Here's how the part is built. I have some questions about the finished solid (model axes, mm). Face numbers are marked on the shaded views. A direction names the side the tool comes from. Give positions to 0.01 mm unless a question says otherwise; leave off trailing zeros. Write each loop counter-clockwise with the first axis right and the second up, starting at its lowest first coordinate (ties: lowest second). Pieces come first, ordered by that corner, then holes. Notation, with made-up numbers: (-27.5, 60.5) - (27.5, 60.5) arc R21 cw to (27.5, 96.5) - close; hole circle Ø5 at (-4, -33.5). An arc over 180 degrees is marked (long way). Use a Markdown table: item, result.
```python
from build123d import *

# Parameters (mm, degrees)
SKETCH2_W           = 115
SKETCH2_H           = 95
BOSS_EXTRUDE1_DEPTH = 5
SKETCH3_W           = 62
SKETCH3_H           = 4
BOSS_EXTRUDE2_DEPTH = 44
RIB1_REACH          = 135.725
SKETCH5_WALL_W      = 295.338836254
SKETCH5_WALL_H      = 8
RIB2_START          = -8
RIB2_DEPTH          = 8
RIB6_REACH          = 135.725
SKETCH7_WALL_W      = 295.32906057
SKETCH7_WALL_H      = 8
BOSS_EXTRUDE3_DEPTH = 8
SKETCH11_R          = 13
SKETCH11_R_2        = 2.1
CUT_EXTRUDE1_DEPTH  = 4
SKETCH12_R          = 13
SKETCH12_R_2        = 2.1
CUT_EXTRUDE2_DEPTH  = 4
SKETCH13_R          = 2.6
CUT_EXTRUDE3_DEPTH  = 5


# Read off the part's stored shape, not the designer's step: Rib2
with BuildPart() as part:
    # Sketch2 → Boss-Extrude1 (new body)
    with BuildSketch(Plane(origin=(0, 0, 0), x_dir=(1, 0, 0), z_dir=(0, 1, 0))):
        Rectangle(SKETCH2_W, SKETCH2_H)
    extrude(amount=BOSS_EXTRUDE1_DEPTH)

    # Sketch3 → Boss-Extrude2 (add)
    with BuildSketch(Plane(origin=(0, 5, 0), x_dir=(1, 0, 0), z_dir=(0, 1, 0))):
        with Locations((-26.5, 45.5)):
            Rectangle(SKETCH3_W, SKETCH3_H)
        with Locations((26.5, -45.5)):
            Rectangle(SKETCH3_W, SKETCH3_H)
    extrude(amount=BOSS_EXTRUDE2_DEPTH)

    # Sketch5 wall → Rib1 (add, up to next)
    with BuildSketch(Plane(origin=(57.5, 14.153417974, 34.346582025), x_dir=(0, -0.707106781187, -0.707106781187), z_dir=(0, 0.707106781187, -0.707106781187)), mode=Mode.PRIVATE) as rib1_sk1:
        with Locations((0, 4)):
            Rectangle(SKETCH5_WALL_W, SKETCH5_WALL_H)
    rib1_tool1 = extrude(rib1_sk1.sketch, amount=-RIB1_REACH, mode=Mode.PRIVATE) - part.part
    add(rib1_tool1.solids().sort_by_distance((57.5, 14.153417974, 34.346582025))[0])

    # Rib2 outline → Rib2 (add)
    with BuildSketch(Plane.ZY.offset(4.5).offset(RIB2_START)):
        Polygon((43.5, 23.306835949), (25.193164051, 5), (43.5, 5), align=None)
    extrude(amount=RIB2_DEPTH)

    # Sketch7 wall → Rib6 (add, up to next)
    with BuildSketch(Plane(origin=(-57.5, 14.149961749, -34.350038251), x_dir=(0, -0.707106781187, 0.707106781187), z_dir=(0, 0.707106781187, 0.707106781187)), mode=Mode.PRIVATE) as rib6_sk1:
        with Locations((0, 4)):
            Rectangle(SKETCH7_WALL_W, SKETCH7_WALL_H)
    rib6_tool1 = extrude(rib6_sk1.sketch, amount=-RIB6_REACH, mode=Mode.PRIVATE) - part.part
    add(rib6_tool1.solids().sort_by_distance((-57.5, 14.149961749, -34.350038251))[0])

    # Sketch9 → Boss-Extrude3 (add)
    with BuildSketch(Plane(origin=(4.5, 0, 0), x_dir=(0, 0, -1), z_dir=(1, 0, 0))):
        Polygon((43.5, 23.299923497), (25.200076503, 5), (43.5, 5), align=None)
    extrude(amount=-BOSS_EXTRUDE3_DEPTH)

    # Sketch11 → Cut-Extrude1 (cut)
    with BuildSketch(Plane(origin=(0, 0, -47.5), x_dir=(-1, 0, 0), z_dir=(0, 0, -1))):
        with Locations((26.5, 27)):
            Circle(SKETCH11_R)
        with Locations((38.874368671, 39.374368671)):
            Circle(SKETCH11_R_2)
        with Locations((38.874368671, 14.625631329)):
            Circle(SKETCH11_R_2)
        with Locations((14.125631329, 14.625631329)):
            Circle(SKETCH11_R_2)
        with Locations((14.125631329, 39.374368671)):
            Circle(SKETCH11_R_2)
    extrude(amount=-CUT_EXTRUDE1_DEPTH, mode=Mode.SUBTRACT)

    # Sketch12 → Cut-Extrude2 (cut)
    with BuildSketch(Plane.XY.offset(47.5)):
        with Locations((26.5, 27)):
            Circle(SKETCH12_R)
        with Locations((38.874368671, 39.374368671)):
            Circle(SKETCH12_R_2)
        with Locations((38.874368671, 14.625631329)):
            Circle(SKETCH12_R_2)
        with Locations((14.125631329, 14.625631329)):
            Circle(SKETCH12_R_2)
        with Locations((14.125631329, 39.374368671)):
            Circle(SKETCH12_R_2)
    extrude(amount=-CUT_EXTRUDE2_DEPTH, mode=Mode.SUBTRACT)

    # Sketch13 → Cut-Extrude3 (cut)
    with BuildSketch(Plane(origin=(0, 5, 0), x_dir=(1, 0, 0), z_dir=(0, 1, 0))):
        with Locations(Location((0, 0, 0), (0, 0, 270))):
            Circle(SKETCH13_R)
        with Locations(Location((52, 0, 0), (0, 0, 270))):
            Circle(SKETCH13_R)
        with Locations(Location((-52, 0, 0), (0, 0, 90))):
            Circle(SKETCH13_R)
    extrude(amount=-CUT_EXTRUDE3_DEPTH, mode=Mode.SUBTRACT)


solid = part.part
```
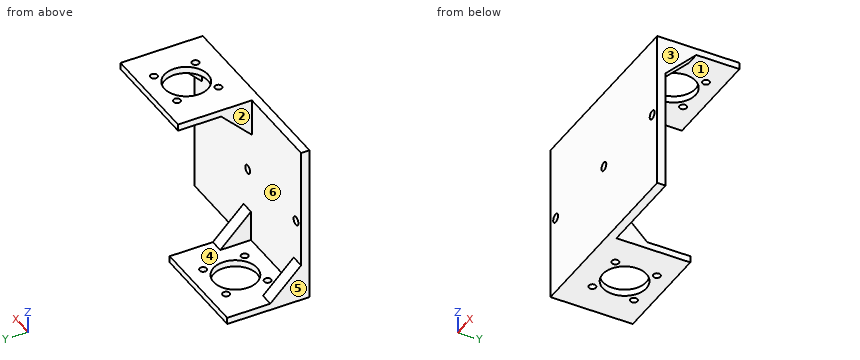
Item 1: If we section it at C-C, the plane x = -26.5: Write out the boundary of the cut face in (y, z), plus the area to 3 significant figures.
Values:
| item | result |
|---|---|
| outline | (0, -47.5) - (14, -47.5) - (14, -43.5) - (5, -43.5) - (5, 47.5) - (0, 47.5) - close; (40, -47.5) - (49, -47.5) - (49, -43.5) - (40, -43.5) - close |
| area | 547 mm2 |
Item 2: For the marked faces 5 and 6, which set-ups out of +Z, -Z, +X, -X, +Y, -Y let a thin tool reach every point of the face, with its end or its side?
Values:
| item | result |
|---|---|
| face 5 | +Z, -Z, -X, +Y, -Y |
| face 6 | +Y |
Item 3: I need wall thicknesses on line 1 along Z through (x, y) = (3, 27); line 2 along Y through (x, z) = (-26, -45); line 3 along X through (y, z) = (10, 32.5). Which ranges of each line are inside material? Lowest first, please. Write a range as [from, to].
Values:
| item | result |
|---|---|
| line 1 | z = [-47.5, -43.5], [43.5, 47.5] |
| line 2 | y = [0, 14.01], [39.99, 49] |
| line 3 | x = [-4.5, 3.5], [49.5, 57.5] |
Item 4: If we section it at B-B, the plane z = 0: Write out the boundary of the cut face in (x, y), plus the area to 3 significant figures.
Values:
| item | result |
|---|---|
| outline | (-57.5, 0) - (-54.6, 0) - (-54.6, 5) - (-57.5, 5) - close; (-49.4, 0) - (-2.6, 0) - (-2.6, 5) - (-49.4, 5) - close; (2.6, 0) - (49.4, 0) - (49.4, 5) - (2.6, 5) - close; (54.6, 0) - (57.5, 0) - (57.5, 5) - (54.6, 5) - close |
| area | 497 mm2 |
Item 5: If we section it at A-A, the plane x = 52: Write out the boundary of the cut face in (y, z).
Values:
| item | result |
|---|---|
| outline | (0, -47.5) - (5, -47.5) - (5, -2.6) - (0, -2.6) - close; (0, 2.6) - (5, 2.6) - (5, 25.19) - (23.31, 43.5) - (49, 43.5) - (49, 47.5) - (0, 47.5) - close |
Item 6: If we section it at D-D, the plane z = -36.5: Write out the boundary of the cut face in (x, y).
Values:
| item | result |
|---|---|
| outline | (-57.5, 0) - (57.5, 0) - (57.5, 5) - (4.5, 5) - (4.5, 16.3) - (-3.5, 16.3) - (-3.5, 5) - (-49.5, 5) - (-49.5, 16.3) - (-57.5, 16.3) - close |
Item 7: Thinking about a two-plate mould opening in X: for the marked faces 1, 2, 3 and 4, which applies, +X half, -X half, draft (parallel to the pull), parting line (faces both ways), or undercut?
Values:
| item | result |
|---|---|
| face 1 | undercut |
| face 2 | -X half |
| face 3 | +X half |
| face 4 | undercut |
Item 8: Will these pins go through, and if not, where does the flat tip stop? pin 1 Ø4 at (x, z) = (5.5, 16.5) entering from +Y; pin 2 Ø9 at (y, z) = (15, 38.5) entering from -X; pin 3 Ø2.5 at (x, y) = (-38.87, 14.63) entering from +Z; pin 4 Ø5.5 at (y, z) = (14, -38) entering from +X.
Values:
| item | result |
|---|---|
| pin 1 | stops at y = 5 |
| pin 2 | stops at x = -4.5 |
| pin 3 | passes through |
| pin 4 | stops at x = 4.5 |
